Verification items for the finished model (mm, model axes). Face numbers are marked on the shaded views. A direction names the side the tool comes from. Coordinates: 2 decimals unless noted, no trailing zeros. Write each loop counter-clockwise with the first axis right and the second up, starting at its lowest first coordinate (ties: lowest second). Pieces come first, ordered by that corner, then holes. Notation, with made-up numbers: (45.25, 31.25) -> (64.25, 31.25) arc R15 ccw to (64.25, 38.25) -> close; hole circle Ø3 at (-5.5, -17.75). An arc over 180 degrees is marked (long way). Answer in a Markdown table with one row per item.
```python
from build123d import *

# Parameters (mm, degrees)
BOSS_EXTRUDE1_DEPTH = 403.86
CUT_EXTRUDE2_START  = -25.4
CUT_EXTRUDE2_DEPTH  = 353.06
CUT_EXTRUDE5_START  = -19.05
SKETCH3_R           = 22.86
CUT_EXTRUDE5_DEPTH  = 353.06
CUT_EXTRUDE6_START  = -19.05
SKETCH4_R           = 22.86
CUT_EXTRUDE6_DEPTH  = 353.06
SKETCH5_R           = 5.715
CUT_EXTRUDE7_DEPTH  = 76.2


with BuildPart() as part:
    # Sketch1 → Boss-Extrude1 (new body)
    with BuildSketch(Plane.XY):
        with BuildLine():
            Line((-10.998522628, 120.65), (-38.114105889, 167.615567884))
            Line((-38.114105889, 167.615567884), (-115.061446619, 123.19))
            Line((-115.061446619, 123.19), (-76.2, 55.88))
            Line((-76.2, 55.88), (-76.2, 0))
            Line((-76.2, 0), (76.2, 0))
            Line((76.2, 0), (76.2, 55.88))
            Line((76.2, 55.88), (115.061446619, 123.19))
            Line((115.061446619, 123.19), (38.114105889, 167.615567884))
            Line((38.114105889, 167.615567884), (10.998522628, 120.65))
            ThreePointArc((10.998522628, 120.65), (0, 114.3), (-10.998522628, 120.65))
        make_face()
    extrude(amount=BOSS_EXTRUDE1_DEPTH)

    # Sketch2 → Cut-Extrude2 (cut)
    with BuildSketch(Plane.XY.offset(403.86).offset(CUT_EXTRUDE2_START)):
        with BuildLine():
            Line((26.311519178, 45.814017315), (50.8, 31.75))
            Line((50.8, 31.75), (50.8, 0))
            Line((50.8, 0), (-50.8, 0))
            Line((-50.8, 0), (-50.8, 31.75))
            Line((-50.8, 31.75), (-26.311519178, 45.814017315))
            ThreePointArc((-26.311519178, 45.814017315), (0, 52.832), (26.311519178, 45.814017315))
        make_face()
    extrude(amount=-CUT_EXTRUDE2_DEPTH, mode=Mode.SUBTRACT)

    # Sketch3 → Cut-Extrude5 (cut)
    with BuildSketch(Plane(origin=(82.108196401, 142.215567884, 0), x_dir=(0.8660254037844397, -0.4999999999999981, 0), z_dir=(0.4999999999999982, 0.8660254037844398, 0)).offset(CUT_EXTRUDE5_START)):
        with Locations(Location((0, -60.96, 0), (0, 0, 180))):
            Circle(SKETCH3_R)
        with Locations(Location((0, -172.72, 0), (0, 0, 180))):
            Circle(SKETCH3_R)
        with Locations(Location((0, -284.48, 0), (0, 0, 180))):
            Circle(SKETCH3_R)
    extrude(amount=-CUT_EXTRUDE5_DEPTH, mode=Mode.SUBTRACT)

    # Sketch4 → Cut-Extrude6 (cut)
    with BuildSketch(Plane(origin=(-82.108196401, 142.215567884, 0), x_dir=(0.866025403784438, 0.5000000000000011, 0), z_dir=(-0.5000000000000011, 0.8660254037844382, 0)).offset(CUT_EXTRUDE6_START)):
        with Locations(Location((0, -340.36, 0), (0, 0, 180))):
            Circle(SKETCH4_R)
        with Locations(Location((0, -228.6, 0), (0, 0, 180))):
            Circle(SKETCH4_R)
        with Locations(Location((0, -116.84, 0), (0, 0, 180))):
            Circle(SKETCH4_R)
    extrude(amount=-CUT_EXTRUDE6_DEPTH, mode=Mode.SUBTRACT)

    # Sketch5 → Cut-Extrude7 (cut)
    with BuildSketch(Plane.XZ):
        with Locations(Location((-63.5, 12.7, 0), (0, 0, 270))):
            Circle(SKETCH5_R)
        with Locations(Location((63.5, 391.16, 0), (0, 0, 270))):
            Circle(SKETCH5_R)
    extrude(amount=-CUT_EXTRUDE7_DEPTH, mode=Mode.SUBTRACT)


solid = part.part
```
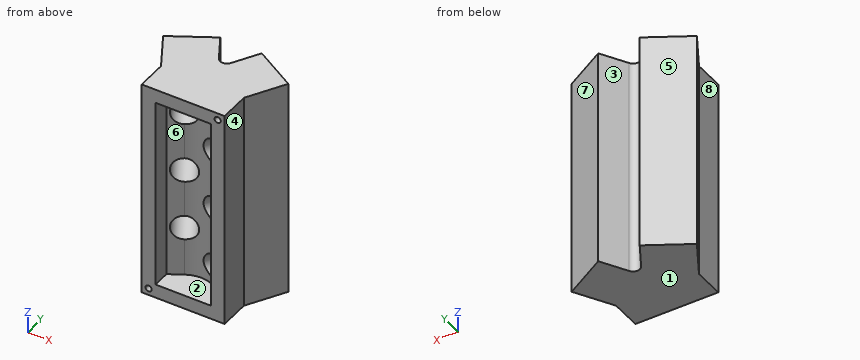
1. Thickness scan on line 1 (Z direction, x = 50, y = 27.5); line 2 (Z direction, x = -63, y = 33); line 3 (X direction, y = 21.5, z = 132). Record the ranges inside material, lowest first. Write a range as from..to.
Geometry says:
| item | result |
|---|---|
| line 1 | 0..25.4, 378.46..403.86 |
| line 2 | 0..7.01, 18.39..403.86 |
| line 3 | -76.2..-50.8, 50.8..76.2 |
2. Depth check by flat-ended pin: P1, Ø10, axis at x = 85.5, z = 284, coming from the +Y side; P2, Ø12, axis at y = 75, z = 227, coming from the +X side; P3, Ø10.5, axis at x = 63.5, z = 391.16, coming from the +Y side. Enter the tip coordinate at first touch or a pass-through.
Geometry says:
| item | result |
|---|---|
| P1 | y = 143.14 |
| P2 | x = 90.7 |
| P3 | y = 155.99 |
3. Mould release check, pull along Z, two halves, no side actions. Record for the marked faces 1, 2 and 3: released by +Z, released by -Z, zero draft, split by the parting line, or undercut.
Geometry says:
| item | result |
|---|---|
| face 1 | released by -Z |
| face 2 | undercut |
| face 3 | zero draft |
4. Section check A-A, the plane z = 12.7. Record the boundary of the cut face in (x, y) (3 decimals), plus the area to 3 significant figures.
Geometry says:
| item | result |
|---|---|
| outline | (-115.061, 123.19) -> (-76.2, 55.88) -> (-76.2, 0) -> (-69.215, 0) -> (-69.215, 76.2) -> (-57.785, 76.2) -> (-57.785, 0) -> (76.2, 0) -> (76.2, 55.88) -> (115.061, 123.19) -> (38.114, 167.616) -> (10.999, 120.65) arc R12.7 cw to (-10.999, 120.65) -> (-38.114, 167.616) -> close |
| area | 24,900 mm^2 |
5. Section check B-B, the plane y = 67. State how many separate pieces and enclosed holes the cut face has, plus the area to 3 significant figures.
Geometry says:
| item | result |
|---|---|
| separate pieces | 1 |
| enclosed holes | 8 |
| area | 55,200 mm^2 |
6. Tool access check on the marked faces 4, 5, 6, 7 and 8. Record the directions out of +Z, -Z, +X, -X, +Y, -Y that give a thin tool (end or side, any length) a straight path to the whole face; none if there is none.
Geometry says:
| item | result |
|---|---|
| face 4 | +Z, -Z, +X, -Y |
| face 5 | +Z, -Z, -X, +Y |
| face 6 | -Y |
| face 7 | +Z, -Z, +X, +Y |
| face 8 | +Z, -Z, -X, -Y |
